```python
from build123d import *

# Parameters (mm, degrees)
BOSS_EXTRU_1_DEPTH      = 50
ESQUISSE2_R             = 1.5
BOSS_EXTRU_2_DEPTH      = 5
ESQUISSE3_R             = 1.25
ENL_V_MAT_EXTRU_1_DEPTH = 10
CHANFREIN1_SIZE         = 0.5


with BuildPart() as part:
    # Esquisse1 → Boss.-Extru.1 (new body)
    with BuildSketch(Plane.XY):
        Polygon((2.5, -1.443375673), (2.5, 1.443375673), (0, 2.886751346), (-2.5, 1.443375673), (-2.5, -1.443375673), (0, -2.886751346), align=None)
    extrude(amount=BOSS_EXTRU_1_DEPTH)

    # Esquisse2 → Boss.-Extru.2 (add)
    with BuildSketch(Plane.XY.offset(50)):
        Circle(ESQUISSE2_R)
    extrude(amount=BOSS_EXTRU_2_DEPTH)

    # Esquisse3 → Enlèv. mat.-Extru.1 (cut)
    with BuildSketch(Plane(origin=(0, 0, 0), x_dir=(-1, 0, 0), z_dir=(0, 0, -1))):
        Circle(ESQUISSE3_R)
    extrude(amount=-ENL_V_MAT_EXTRU_1_DEPTH, mode=Mode.SUBTRACT)

    # Chanfrein1
    chanfrein1_edges = [part.edges().sort_by_distance(p)[0] for p in [
        (-1.5, 0, 55),
    ]]
    chamfer(chanfrein1_edges, length=CHANFREIN1_SIZE)


solid = part.part
```
Geometry check sheet. Reference: the model listing, model coordinates, mm. A direction names the side the tool comes from. Round coordinates to 2 decimals unless told otherwise and drop trailing zeros. Loops run counter-clockwise (first coordinate to the right, second up) from the corner with the lowest first, then second, coordinate; pieces in that order, holes last. Notation, with made-up numbers: (63, -21.75) -> (110, -21.75) arc R15 ccw to (110, -9.75) -> close; hole circle Ø7 at (47, 82.5). An arc over 180 degrees is marked (long way). Use a Markdown table: item, result.
(1) Go/stop test with a flat-tipped pin: P1, Ø2, axis at x = -0.5, y = -2, coming from the +Z side. Record where the tip stops, or that it passes through.
Calculated:
| item | result |
|---|---|
| P1 | z = 54.94 |
(2) Sectioned sample at B-B (z = 47). Enter the section's corners in (x, y), then the cut area to 3 significant figures.
Calculated:
| item | result |
|---|---|
| outline | (-2.5, -1.44) -> (0, -2.89) -> (2.5, -1.44) -> (2.5, 1.44) -> (0, 2.89) -> (-2.5, 1.44) -> close |
| area | 21.7 mm² |
(3) Set-up check for faces 1 (the flat face through (-2.5, 0, 25)), 2 (the cylindrical face through (-1.5, 0.07, 52.22)), 3 (the cylindrical face through (0.27, -1.22, 4.93)): record each of +Z, -Z, +X, -X, +Y, -Y from which the full face is reachable in a straight line by a thin tool's end or side.
Calculated:
| item | result |
|---|---|
| face 1 | +Z, -Z, -X, +Y, -Y |
| face 2 | +Z |
| face 3 | -Z |
(4) Sectioned sample at A-A (y = 0). Enter the section's corners in (x, z), then the cut area to 3 significant figures.
Calculated:
| item | result |
|---|---|
| outline | (-2.5, 0) -> (-1.25, 0) -> (-1.25, 10) -> (1.25, 10) -> (1.25, 0) -> (2.5, 0) -> (2.5, 50) -> (1.5, 50) -> (1.5, 54.5) -> (1, 55) -> (-1, 55) -> (-1.5, 54.5) -> (-1.5, 50) -> (-2.5, 50) -> close |
| area | 240 mm² |
(5) Scan lines: probe 1 along Y at (x, z) = (0, 6); probe 2 along Z at (x, y) = (-0.95, -2.05); probe 3 along Y at (x, z) = (2.05, 22). Record each from-to range of solid material in increasing order.
Calculated:
| item | result |
|---|---|
| probe 1 | -2.89 to -1.25, 1.25 to 2.89 |
| probe 2 | 0 to 50 |
| probe 3 | -1.7 to 1.7 |
(6) Mould release check, pull along X, two halves, no side actions. Record for faces 4 (the flat face through (0, 0, 55)), 5 (the flat face through (0, 0, 10)), 6 (the flat face through (2.5, 0, 25)): released by +X, released by -X, zero draft, split by the parting line, or undercut.
Calculated:
| item | result |
|---|---|
| face 4 | zero draft |
| face 5 | undercut |
| face 6 | released by +X |
